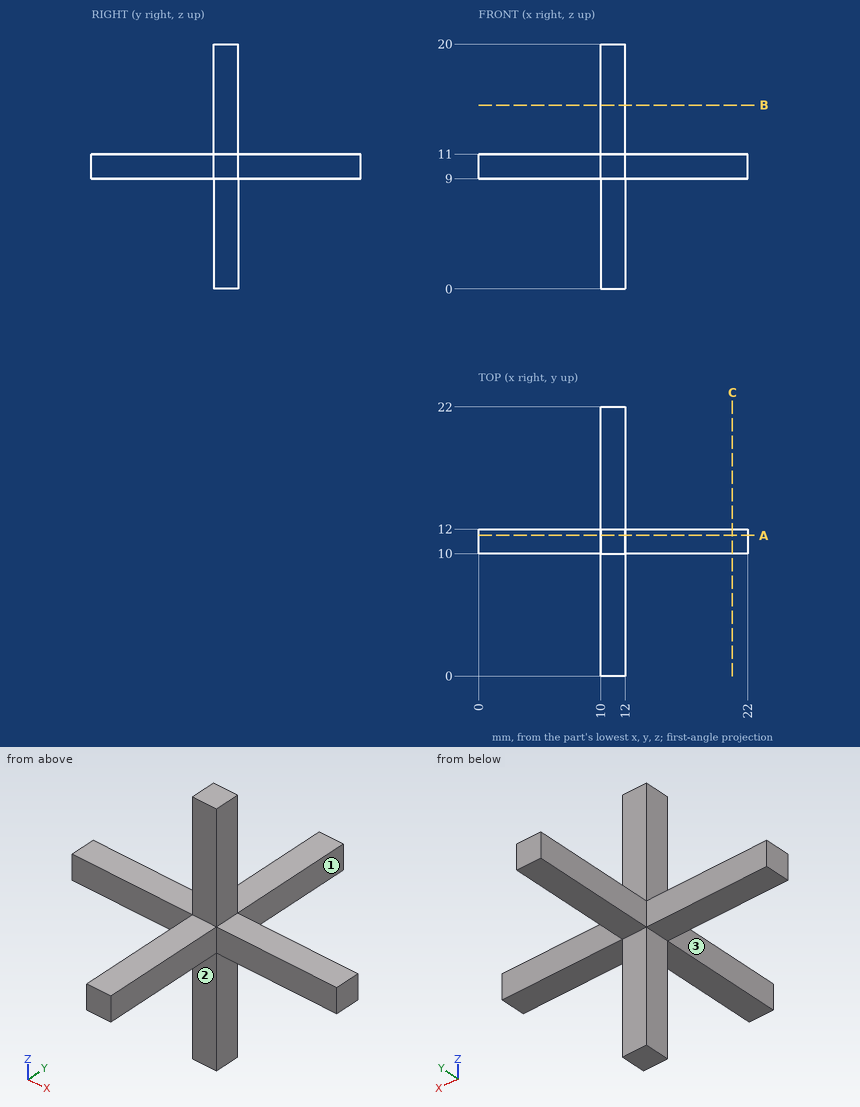
Print and shaded views of the part. All mm, measured from the part's lowest x, y and z. A direction names the side the tool comes from. Round coordinates to 2 decimals unless told otherwise and drop trailing zeros. Write each loop counter-clockwise with the first axis right and the second up, starting at its lowest first coordinate (ties: lowest second). Pieces come first, ordered by that corner, then holes.
(1) Slice it at C-C, the plane x = 20.75. Write the cut outline in (y, z), and give its area (3 significant figures).
(2) 3-axis set-ups, long thin cutter, end or side, ignore diameter. For the marked faces 1, 2 and 3: which of +Z, -Z, +X, -X, +Y, -Y reach the whole face in a straight line?
(3) Slice it at B-B, the plane z = 15. Write the cut outline in (x, y).
(4) Slice it at A-A, the plane y = 11.5. Write the cut outline in (x, z), and give its area (3 significant figures).
(5) Drop flat-ended pins along their axis: P1, Ø1.6, axis at y = 16.5, z = 10, coming from the -X side; P2, Ø2, axis at x = 10, y = 16, coming from the +Z side; P3, Ø1, axis at x = 11, y = 18.5, coming from the -Z side. Give the stop position or say it passes through.
(6) Probe line 1 along X through (y, z) = (11.5, 15); line 2 along Z through (x, y) = (11.75, 18.75). List the from-to ranges inside material, lowest first.
From the geometry:
1. outline: (10, 9) - (12, 9) - (12, 11) - (10, 11) - close
1. area: 4.00 mm2
2. face 1: +Z, -Z, +X, +Y
2. face 2: -Z, +X, -X, -Y
2. face 3: +Z, -Z, -X, -Y
3. outline: (10, 10) - (12, 10) - (12, 12) - (10, 12) - close
4. outline: (0, 9) - (10, 9) - (10, 0) - (12, 0) - (12, 9) - (22, 9) - (22, 11) - (12, 11) - (12, 20) - (10, 20) - (10, 11) - (0, 11) - close
4. area: 80.0 mm2
5. P1: stops at x = 10
5. P2: stops at z = 11
5. P3: stops at z = 9
6. line 1: x = 10 to 12
6. line 2: z = 9 to 11
